Build history of the part. All positions in model axes, mm. Face numbers are marked on the shaded views. A direction names the side the tool comes from. Give positions to 0.01 mm unless a question says otherwise; leave off trailing zeros. Write each loop counter-clockwise with the first axis right and the second up, starting at its lowest first coordinate (ties: lowest second). Pieces come first, ordered by that corner, then holes. Notation, with made-up numbers: (19, 37) -> (53, 37) arc R27 cw to (53, 66) -> close; hole circle Ø8 at (29.5, 89.5). An arc over 180 degrees is marked (long way). Write item = value, one per line. Start each with the question number.
Q1. Saw through at C-C, the plane z = 14. Give the number of separate pieces and of enclosed holes in the cut face, then the cut area to 3 significant figures.
Q2. Drop flat-ended pins along their axis: P1, Ø8, axis at x = -34, z = 4, coming from the +Y side; P2, Ø2, axis at y = 4, z = 12.5, coming from the +X side; P3, Ø0.9, axis at y = 4, z = 13, coming from the +X side. Give the stop position or say it passes through.
Q3. Saw through at A-A, the plane z = 21.5. List the corners of the cut face in (x, y), then the cut area to 3 significant figures.
Q4. Saw through at B-B, the plane x = -16. List the corners of the cut face in (y, z).
Q5. Wall check: line 1 (X direction, y = 6.75, z = 22.5); line 2 (Z direction, x = -11, y = 7.25); line 3 (Y direction, x = -40.5, z = 0.5). Give the ranges that are in metal, low to high.
Q6. Mould opens along Y. For the marked faces 3, 4, 5 and 6 say: pulls with the +Y half, pulls with the -Y half, needs draft (parallel to the pull), parting line crosses it, or undercut.
Q7. Tool access for the marked faces 1 and 2: list every direction of +Z, -Z, +X, -X, +Y, -Y with a clear straight run to the whole face (end or side of a thin tool).
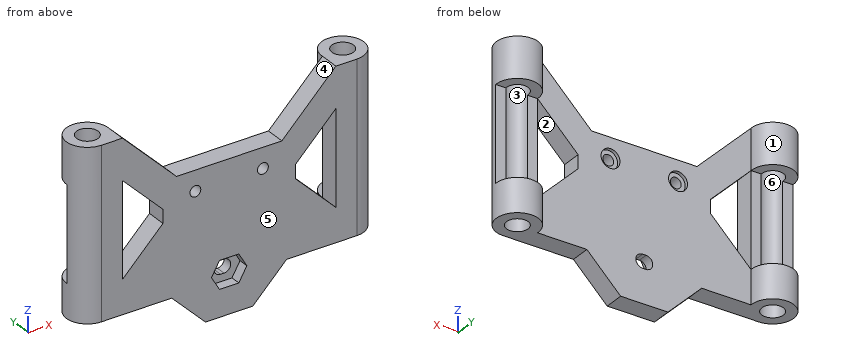
from build123d import *

# Parameters (mm, degrees)
SKETCH_1_R           = 3.1
SKETCH_1_R_2         = 1.6
EXTRUDE_1_DEPTH      = 25
EXTRUDE_2_DEPTH      = 2.945
CUT_EXTRUDE_1_DEPTH  = 56.771287036
CUT_EXTRUDE_START    = -1.5
CUT_EXTRUDE_4_DEPTH  = 1.5
SKETCH_6_R           = 0.8
CUT_EXTRUDE_5_DEPTH  = 56.771287036
CUT_EXTRUDE_6_DEPTH  = 56.771287036
SKETCH_9_W           = 14
SKETCH_9_H           = 3.255
CUT_EXTRUDE_9_DEPTH  = 47.133536551
SKETCH_10_R          = 1.4
CUT_EXTRUDE_11_DEPTH = 0.5


with BuildPart() as part:
    # 草图1 → 凸台-拉伸1 (new body)
    # profile 1 of 3: a face of its own
    with BuildSketch(Plane.XY):
        with Locations((-46.647778168, 5.529205914)):
            Circle(SKETCH_1_R)
        with Locations((-46.647778168, 5.529205914)):
            Circle(SKETCH_1_R_2, mode=Mode.SUBTRACT)
    # profile 2 of 3: a face of its own
    with BuildSketch(Plane.XY):
        with BuildLine():
            ThreePointArc((-43.551655593, 5.374205914), (-44.511250611, 3.283042519), (-46.647778168, 2.429205914))
            Line((-46.647778168, 2.429205914), (-8.847778168, 2.429205914))
            ThreePointArc((-8.847778168, 2.429205914), (-10.984305724, 3.283042519), (-11.943900743, 5.374205914))
            Line((-11.943900743, 5.374205914), (-43.551655593, 5.374205914))
        make_face()
    # profile 3 of 3: a face of its own
    with BuildSketch(Plane.XY):
        with Locations((-8.847778168, 5.529205914)):
            Circle(SKETCH_1_R)
        with Locations((-8.847778168, 5.529205914)):
            Circle(SKETCH_1_R_2, mode=Mode.SUBTRACT)
    extrude(amount=EXTRUDE_1_DEPTH)

    # 草图2 → 凸台-拉伸2 (add)
    with BuildSketch(Plane(origin=(0, 5.374205914, 0), x_dir=(1, 0, 0), z_dir=(0, 1, 0))):
        Polygon((-19.247778168, 0), (-24.247778168, 5), (-31.247778168, 5), (-36.247778168, 0), align=None)
    extrude(amount=-EXTRUDE_2_DEPTH)

    # 草图3 → 切除-拉伸1 (cut, through all)
    with BuildSketch(Plane(origin=(0, 5.374205914, 0), x_dir=(1, 0, 0), z_dir=(0, 1, 0))):
        with BuildLine():
            Line((-27.997778168, 0), (-27.497778168, 0))
            ThreePointArc((-27.497778168, 0), (-26.497778168, -1), (-27.497778168, -2))
            Line((-27.497778168, -2), (-27.997778168, -2))
            ThreePointArc((-27.997778168, -2), (-28.997778168, -1), (-27.997778168, 0))
        make_face()
    extrude(amount=-CUT_EXTRUDE_1_DEPTH, mode=Mode.SUBTRACT)

    # 草图5 → 切除-拉伸4 (cut)
    # profile 1 of 3: a face of its own
    with BuildSketch(Plane(origin=(0, 2.429205914, 0), x_dir=(-1, 0, 0), z_dir=(0, -1, 0)).offset(CUT_EXTRUDE_START)):
        Polygon((25.630642064, -1), (26.814210116, 1.05), (26.314210116, 1.05), (25.130642064, -1), (26.314210116, -3.05), (26.814210116, -3.05), align=None)
    # profile 2 of 3: a face of its own
    with BuildSketch(Plane(origin=(0, 2.429205914, 0), x_dir=(-1, 0, 0), z_dir=(0, -1, 0)).offset(CUT_EXTRUDE_START)):
        Polygon((28.68134622, -3.05), (29.864914271, -1), (28.68134622, 1.05), (26.814210116, 1.05), (25.630642064, -1), (26.814210116, -3.05), align=None)
        with BuildLine():
            ThreePointArc((27.497778168, -2), (26.497778168, -1), (27.497778168, 0))
            Line((27.497778168, 0), (27.997778168, 0))
            ThreePointArc((27.997778168, 0), (28.997778168, -1), (27.997778168, -2))
            Line((27.997778168, -2), (27.497778168, -2))
        make_face(mode=Mode.SUBTRACT)
    # profile 3 of 3: a face of its own
    with BuildSketch(Plane(origin=(0, 2.429205914, 0), x_dir=(-1, 0, 0), z_dir=(0, -1, 0)).offset(CUT_EXTRUDE_START)):
        Polygon((28.68134622, 1.05), (29.864914271, -1), (28.68134622, -3.05), (29.18134622, -3.05), (30.364914271, -1), (29.18134622, 1.05), align=None)
    extrude(amount=CUT_EXTRUDE_4_DEPTH, mode=Mode.SUBTRACT)

    # 草图6 → 切除-拉伸5 (cut, through all)
    with BuildSketch(Plane(origin=(0, 5.374205914, 0), x_dir=(1, 0, 0), z_dir=(0, 1, 0))):
        with Locations(Location((-32.747778168, -14, 0), (0, 0, 270))):
            Circle(SKETCH_6_R)
        with Locations(Location((-22.747778168, -14, 0), (0, 0, 270))):
            Circle(SKETCH_6_R)
    extrude(amount=-CUT_EXTRUDE_5_DEPTH, mode=Mode.SUBTRACT)

    # 草图7 → 切除-拉伸6 (cut, through all)
    with BuildSketch(Plane(origin=(0, 5.374205914, 0), x_dir=(1, 0, 0), z_dir=(0, 1, 0))):
        Polygon((-35.547778168, -17), (-43.547778168, -25), (-11.943900743, -25), (-19.943900743, -17), align=None)
        Polygon((-37.547778168, -13), (-37.547778168, -11), (-43.547778168, -5), (-43.547778168, -19), align=None)
        Polygon((-11.947778168, -5), (-17.947778168, -11), (-17.947778168, -13), (-11.947778168, -19), align=None)
    extrude(amount=-CUT_EXTRUDE_6_DEPTH, mode=Mode.SUBTRACT)

    # 草图9 → 切除-拉伸9 (cut, through all)
    with BuildSketch(Plane.ZY.offset(11.947778168)):
        with Locations((12, 7.001705914)):
            Rectangle(SKETCH_9_W, SKETCH_9_H)
    cut_extrude_9 = extrude(amount=-CUT_EXTRUDE_9_DEPTH, mode=Mode.SUBTRACT)

    # 镜向1: 切除-拉伸9 across plane
    add(cut_extrude_9.mirror(Plane(origin=(-27.747778168, 0, 0), x_dir=(0, 0, 1), z_dir=(1, 0, 0))), mode=Mode.SUBTRACT)

    # 草图10 → 切除-拉伸11 (cut)
    with BuildSketch(Plane(origin=(0, 5.374205914, 0), x_dir=(1, 0, 0), z_dir=(0, 1, 0))):
        with Locations(Location((-22.747778168, -14, 0), (0, 0, 270))):
            Circle(SKETCH_10_R)
        with Locations(Location((-32.747778168, -14, 0), (0, 0, 270))):
            Circle(SKETCH_10_R)
    extrude(amount=-CUT_EXTRUDE_11_DEPTH, mode=Mode.SUBTRACT)


solid = part.part
Report:
q1.separate_pieces = 5
q1.enclosed_holes = 0
q1.area = 78.3 mm2
q2.P1 = 5.37
q2.P2 = -5.79
q2.P3 = -5.94
q3.outline = (-46.65, 2.43) -> (-40.05, 2.43) -> (-40.05, 5.37) -> (-43.55, 5.37) arc R3.1 ccw (long way) to start; (-15.44, 2.43) -> (-8.85, 2.43) arc R3.1 ccw (long way) to (-11.94, 5.37) -> (-15.44, 5.37) -> close; hole circle Ø3.2 at (-46.65, 5.53); hole circle Ø3.2 at (-8.85, 5.53)
q3.area = 69.0 mm2
q4.outline = (2.43, 0) -> (5.37, 0) -> (5.37, 9.05) -> (2.43, 9.05) -> close; (2.43, 14.95) -> (5.37, 14.95) -> (5.37, 20.94) -> (2.43, 20.94) -> close
q5.line_1 = -49.5 to -47.68, -45.61 to -43.8, -11.7 to -9.88, -7.81 to -6
q5.line_2 = 0 to 5, 19 to 25
q5.line_3 = 2.43 to 5.37
q6.face_3 = undercut
q6.face_4 = needs draft
q6.face_5 = pulls with the -Y half
q6.face_6 = undercut
q7.face_1 = +Z, -Z
q7.face_2 = +Y, -Y
